Source: three-view drawing plus pictorial views. Frame: mm from the lowest corner of the part. Give positions to 0.01 mm unless a question says otherwise; leave off trailing zeros. Write each loop counter-clockwise with the first axis right and the second up, starting at its lowest first coordinate (ties: lowest second). Pieces come first, ordered by that corner, then holes. Notation, with made-up numbers: (1, 84) -> (35, 84) arc R14 ccw to (35, 109) -> close; hole circle Ø6 at (-35, 46). An arc over 180 degrees is marked (long way). Write item = value, one per line.
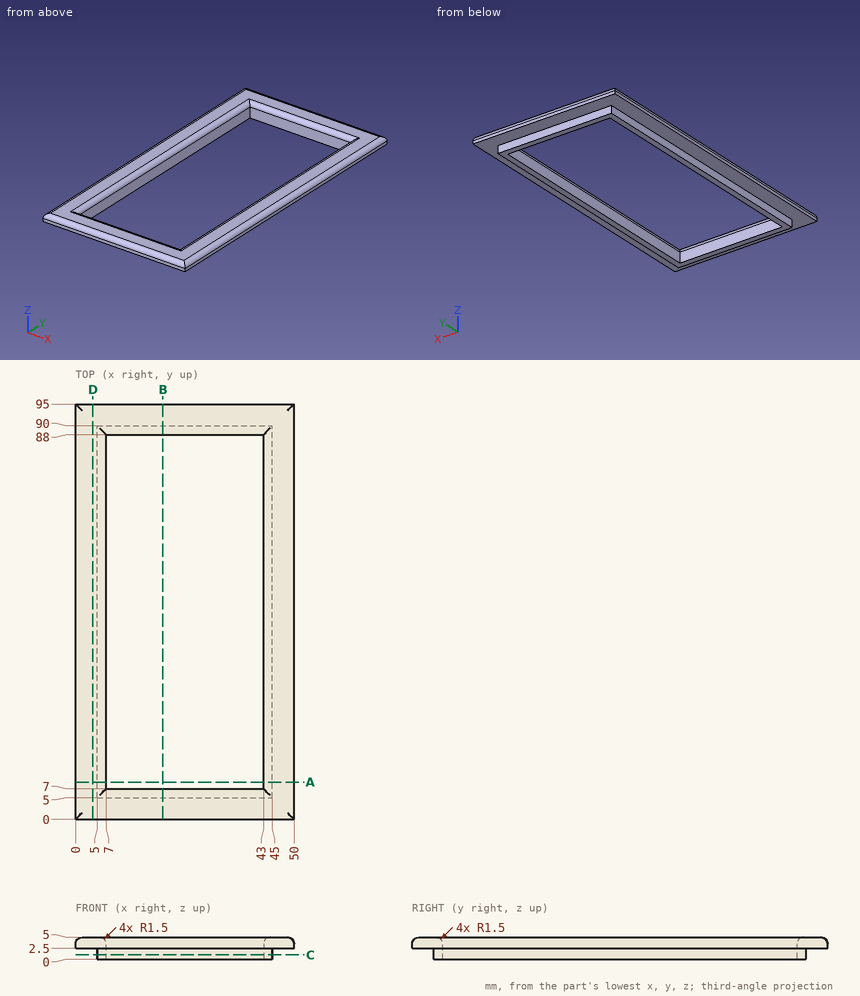
1) Cut plane A-A (y = 8.5). Return the cut outline in (x, z), then the cut area to 3 significant figures.
Computed:
outline = (0, 2.5) -> (5, 2.5) -> (5, 0) -> (7, 0) -> (7, 3.5) arc R1.5 ccw to (5.5, 5) -> (1.5, 5) arc R1.5 ccw to (0, 3.5) -> close; (43, 0) -> (45, 0) -> (45, 2.5) -> (50, 2.5) -> (50, 3.5) arc R1.5 ccw to (48.5, 5) -> (44.5, 5) arc R1.5 ccw to (43, 3.5) -> close
area = 43.1 mm²
2) Cut plane B-B (x = 20). Return the cut outline in (y, z), then the cut area to 3 significant figures.
Computed:
outline = (0, 2.5) -> (5, 2.5) -> (5, 0) -> (7, 0) -> (7, 3.5) arc R1.5 ccw to (5.5, 5) -> (1.5, 5) arc R1.5 ccw to (0, 3.5) -> close; (88, 0) -> (90, 0) -> (90, 2.5) -> (95, 2.5) -> (95, 3.5) arc R1.5 ccw to (93.5, 5) -> (89.5, 5) arc R1.5 ccw to (88, 3.5) -> close
area = 43.1 mm²
3) Cut plane D-D (x = 4). Return the cut outline in (y, z), then the cut area to 3 significant figures.
Computed:
outline = (0, 2.5) -> (95, 2.5) -> (95, 3.5) arc R1.5 ccw to (93.5, 5) -> (1.5, 5) arc R1.5 ccw to (0, 3.5) -> close
area = 237 mm²
4) Contact query for flat-ended pins moving along their axis: pin 1 (1.8 mm diameter, centred on y = 48, z = 1.5, fed in from +X); pin 2 (1.8 mm diameter, centred on x = 27.5, z = 1, fed in from +Y); pin 3 (0.8 mm diameter, centred on x = 32, z = 1.5, fed in from -Y). Output: stop coordinate, or through.
Computed:
pin_1 = 45
pin_2 = 90
pin_3 = 5
5) Material intervals for L1, parallel to X at y = 60, z = 3.65; L2, parallel to X at y = 65.5, z = 0.4; L3, parallel to Y at x = 11, z = 2.55, sorted ascending.
Computed:
L1 = 0.01 to 6.99, 43.01 to 49.99
L2 = 5 to 7, 43 to 45
L3 = 0 to 7, 88 to 95
6) Cut plane C-C (z = 1). Return the cut outline in (x, y).
Computed:
outline = (5, 5) -> (45, 5) -> (45, 90) -> (5, 90) -> close; hole (7, 7) -> (43, 7) -> (43, 88) -> (7, 88) -> close
